Source: CAD feature listing. Evaluate the final solid. Frame: model axes, mm. A direction names the side the tool comes from. Coordinates: 2 decimals unless noted, no trailing zeros. Order: outer loops, then holes, each group sorted by start corner. A loop starts at its lowest first (then second) coordinate and runs counter-clockwise, first axis right, second up.
Item 1: Section A-A on z = 0. Return the cut outline in (x, y), then the cut area to 3 significant figures.
Item 2: Mould query, pull axis X, two halves, no side actions, for faces 1 (the flat face through (-23.43, 0, -7.73)), 2 (the cylindrical face through (-29.23, 23.15, -6.49)), 3 (the conical face through (24.57, 15.28, -3.23)). Classes: released by +X, released by -X, zero draft, split by the parting line, or undercut.
Item 3: Section D-D on y = 17.5. Return the cut outline in (x, z), then the cut area to 3 significant figures.
Item 4: Ray query, line 1 (X direction, y = 5, z = 0); line 2 (X direction, y = 22.25, z = 0); line 3 (Y direction, x = 8.5, z = -7). Return the intervals inside material, ascending.
Item 5: Contact query for flat-ended pins moving along their axis: P1, Ø5, axis at y = 24.5, z = 6.5, coming from the +X side; P2, Ø6, axis at x = 4.5, y = 20.5, coming from the +Z side; P3, Ø1, axis at y = 26, z = -22.5, coming from the +X side. Output: stop coordinate, or through.
Item 6: Reachability of faces 4 (the flat face through (0, 29, 0)), 5 (the flat face through (0, 30, 0)), 6 (the cylindrical face through (22.345, 7.605, 14.246)) from +Z, -Z, +X, -X, +Y, -Y: full face, straight path, thin tool, end or side. Return the list, or none.
Item 7: Section B-B on x = 0. Return the cut outline in (y, z), then the cut area to 3 significant figures.
Item 8: Section C-C on y = 2. Return the cut outline in (x, z), then the cut area to 3 significant figures.
from build123d import *

# Parameters (mm, degrees)
F0_W = 15
F0_H = 2


with BuildPart() as f1:
    # F0 (on Right) → F1 (revolve)
    with BuildSketch(Plane.YZ):
        with Locations((7.5, 25.5)):
            Rectangle(F0_W, F0_H)
        Polygon((15, 26.5), (15, 24.5), (19.44, 28.94), (17.44, 28.94), align=None)
        Polygon((17.44, 28.94), (19.44, 28.94), (20.44, 29.94), (18.44, 29.94), align=None)
        with BuildLine():
            Line((29, 26.94), (29, 0))
            Line((29, 0), (30, 0))
            Line((30, 0), (30, 27.94))
            ThreePointArc((30, 27.94), (29.4142135624, 29.3542135624), (28, 29.94))
            Line((28, 29.94), (20.44, 29.94))
            Line((20.44, 29.94), (19.44, 28.94))
            Line((19.44, 28.94), (27, 28.94))
            ThreePointArc((27, 28.94), (28.4142135624, 28.3542135624), (29, 26.94))
        make_face()
    revolve(axis=Axis((0, 7.5, 0), (0, 1, 0)))


solid = f1.part
Answer list:
1. outline: (-29.94, 18.44) - (-26.5, 15) - (-26.5, 0) - (-24.5, 0) - (-24.5, 15) - (-28.94, 19.44) - (-28.94, 27) arc R2 cw to (-26.94, 29) - (26.94, 29) arc R2 cw to (28.94, 27) - (28.94, 19.44) - (24.5, 15) - (24.5, 0) - (26.5, 0) - (26.5, 15) - (29.94, 18.44) - (29.94, 28) arc R2 ccw to (27.94, 30) - (-27.94, 30) arc R2 ccw to (-29.94, 28) - close
1. area: 156 mm2
2. face 1: zero draft
2. face 2: split by the parting line
2. face 3: undercut
3. outline: circle Ø58 at (0, 0); hole circle Ø54 at (0, 0)
3. area: 352 mm2
4. line 1: x = -26.5 to -24.5, 24.5 to 26.5
4. line 2: x = -29.94 to -28.94, 28.94 to 29.94
4. line 3: y = 29 to 30
5. P1: stops at x = 29.67
5. P2: stops at z = 29.9
5. P3: stops at x = 20.31
6. face 4: none
6. face 5: +Z, -Z, +X, -X, +Y
6. face 6: -Y
7. outline: (0, -26.5) - (15, -26.5) - (18.44, -29.94) - (28, -29.94) arc R2 ccw to (30, -27.94) - (30, 27.94) arc R2 ccw to (28, 29.94) - (18.44, 29.94) - (15, 26.5) - (0, 26.5) - (0, 24.5) - (15, 24.5) - (19.44, 28.94) - (27, 28.94) arc R2 cw to (29, 26.94) - (29, -26.94) arc R2 cw to (27, -28.94) - (19.44, -28.94) - (15, -24.5) - (0, -24.5) - close
7. area: 156 mm2
8. outline: circle Ø53 at (0, 0); hole circle Ø49 at (0, 0)
8. area: 320 mm2
